Geometry check sheet. Reference: drawing and pictorial views, mm from the part's lowest x, y, z. A direction names the side the tool comes from. Give positions to 0.01 mm unless a question says otherwise; leave off trailing zeros. Loops run counter-clockwise (first coordinate to the right, second up) from the corner with the lowest first, then second, coordinate; pieces in that order, holes last. Notation, with made-up numbers: (40, 47.5) - (61, 47.5) arc R18 cw to (61, 60.5) - close; hole circle Ø6 at (75, 82.5). An arc over 180 degrees is marked (long way). Use CSV: the item, a comma, the result in double quotes.
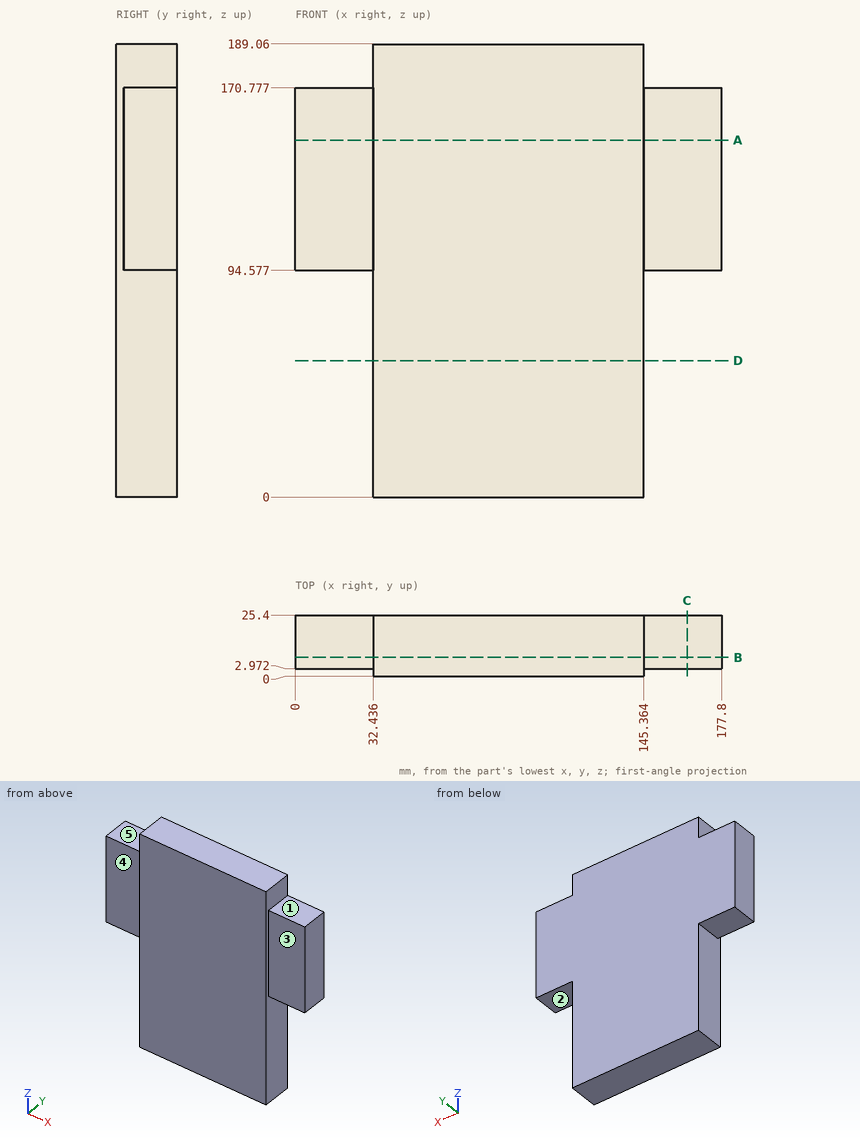
1. Sectioned sample at B-B, the plane y = 7.75. Record the boundary of the cut face in (x, z) (1 decimal), and give its area (3 significant figures).
Completed:
outline,"(0, 94.6) - (32.4, 94.6) - (32.4, 0) - (145.4, 0) - (145.4, 94.6) - (177.8, 94.6) - (177.8, 170.8) - (145.4, 170.8) - (145.4, 189.1) - (32.4, 189.1) - (32.4, 170.8) - (0, 170.8) - close"
area,"26,300 mm²"
2. Sectioned sample at D-D, the plane z = 57. Record the boundary of the cut face in (x, y) (1 decimal), and give its area (3 significant figures).
Completed:
outline,"(32.4, 0) - (145.4, 0) - (145.4, 25.4) - (32.4, 25.4) - close"
area,"2,870 mm²"
3. Scan lines: line 1 along X through (y, z) = (16.5, 92) (1 decimal); line 2 along Z through (x, y) = (145.5, 5.5); line 3 along Y through (x, z) = (20, 161). Record each from-to range of solid material in increasing order.
Completed:
line 1,"x = 32.4 to 145.4"
line 2,"z = 94.58 to 170.78"
line 3,"y = 2.97 to 25.4"
4. Sectioned sample at A-A, the plane z = 149. Record the boundary of the cut face in (x, y) (1 decimal).
Completed:
outline,"(0, 3) - (32.4, 3) - (32.4, 0) - (145.4, 0) - (145.4, 3) - (177.8, 3) - (177.8, 25.4) - (0, 25.4) - close"
5. Set-up check for the marked faces 1, 2, 3, 4 and 5: record each of +Z, -Z, +X, -X, +Y, -Y from which the full face is reachable in a straight line by a thin tool's end or side.
Completed:
face 1,"+Z, +X, +Y, -Y"
face 2,"-Z, +X, +Y, -Y"
face 3,"+Z, -Z, +X, -Y"
face 4,"+Z, -Z, -X, -Y"
face 5,"+Z, -X, +Y, -Y"
6. Sectioned sample at C-C, the plane x = 163.5. Record the boundary of the cut face in (y, z), and give its area (3 significant figures).
Completed:
outline,"(2.97, 94.58) - (25.4, 94.58) - (25.4, 170.78) - (2.97, 170.78) - close"
area,"1,710 mm²"
7. Go/stop test with flat-tipped pins: pin 1 Ø11 at (x, y) = (9.5, 9.5) entering from -Z; pin 2 Ø10 at (y, z) = (18, 68) entering from -X; pin 3 Ø5 at (x, z) = (155, 146) entering from -Y; pin 4 Ø6 at (x, z) = (28, 47.5) entering from +Y. Record where each tip stops, or that it passes through.
Completed:
pin 1,"stops at z = 94.58"
pin 2,"stops at x = 32.44"
pin 3,"stops at y = 2.97"
pin 4,"passes through"
